Model file for the job. Use its own axes, mm. A direction names the side the tool comes from. Round coordinates to 2 decimals unless told otherwise and drop trailing zeros. Loops run counter-clockwise (first coordinate to the right, second up) from the corner with the lowest first, then second, coordinate; pieces in that order, holes last. Notation, with made-up numbers: (-19, -7.5) - (14, -7.5) arc R30 cw to (14, 20.5) - close; hole circle Ø7 at (-13.75, -18.75). An arc over 180 degrees is marked (long way). Use one line per item in the form item = value.
from build123d import *

# Parameters (mm, degrees)
F1_DEPTH       = 7
F0_R           = 2.75
F2_DEPTH       = 3.175
F3_R           = 12.7
F4_DEPTH       = 6.35
F5_D           = 3.3
F5_CBORE_D     = 6.5
F5_CBORE_DEPTH = 2.5
F6_R           = 5.08
F7_R           = 1.27


with BuildPart() as f1:
    # F0 (on Front) → F1 (new body)
    with BuildSketch(Plane.XZ):
        with BuildLine():
            Line((19.05, 0), (-19.05, 0))
            ThreePointArc((-19.05, 0), (-27.0823171118, -4.4056732068), (-27.6841325359, -13.5471114297))
            Line((-27.6841325359, -13.5471114297), (-8.6341325359, -54.4411114297))
            ThreePointArc((-8.6341325359, -54.4411114297), (0, -59.944), (8.6341325359, -54.4411114297))
            Line((8.6341325359, -54.4411114297), (27.6841325359, -13.5471114297))
            ThreePointArc((27.6841325359, -13.5471114297), (27.0823171118, -4.4056732068), (19.05, 0))
        make_face()
        Polygon((4.9074772881, -50.419), (2.4537386441, -54.669), (-2.4537386441, -54.669), (-4.9074772881, -50.419), (-2.4537386441, -46.169), (2.4537386441, -46.169), align=None, mode=Mode.SUBTRACT)
        Polygon((-14.1425227119, -9.525), (-16.5962613559, -13.775), (-21.5037386441, -13.775), (-23.9574772881, -9.525), (-21.5037386441, -5.275), (-16.5962613559, -5.275), align=None, mode=Mode.SUBTRACT)
        Polygon((23.9574772881, -9.525), (21.5037386441, -13.775), (16.5962613559, -13.775), (14.1425227119, -9.525), (16.5962613559, -5.275), (21.5037386441, -5.275), align=None, mode=Mode.SUBTRACT)
    extrude(amount=F1_DEPTH)

    # F0 (on Front) → F2 (join)
    with BuildSketch(Plane.XZ):
        with BuildLine():
            Line((19.05, 0), (-19.05, 0))
            ThreePointArc((-19.05, 0), (-27.0823171118, -4.4056732068), (-27.6841325359, -13.5471114297))
            Line((-27.6841325359, -13.5471114297), (-8.6341325359, -54.4411114297))
            ThreePointArc((-8.6341325359, -54.4411114297), (0, -59.944), (8.6341325359, -54.4411114297))
            Line((8.6341325359, -54.4411114297), (27.6841325359, -13.5471114297))
            ThreePointArc((27.6841325359, -13.5471114297), (27.0823171118, -4.4056732068), (19.05, 0))
        make_face()
        Polygon((4.9074772881, -50.419), (2.4537386441, -54.669), (-2.4537386441, -54.669), (-4.9074772881, -50.419), (-2.4537386441, -46.169), (2.4537386441, -46.169), align=None, mode=Mode.SUBTRACT)
        Polygon((-14.1425227119, -9.525), (-16.5962613559, -13.775), (-21.5037386441, -13.775), (-23.9574772881, -9.525), (-21.5037386441, -5.275), (-16.5962613559, -5.275), align=None, mode=Mode.SUBTRACT)
        Polygon((23.9574772881, -9.525), (21.5037386441, -13.775), (16.5962613559, -13.775), (14.1425227119, -9.525), (16.5962613559, -5.275), (21.5037386441, -5.275), align=None, mode=Mode.SUBTRACT)
        Polygon((16.5962613559, -13.775), (21.5037386441, -13.775), (23.9574772881, -9.525), (21.5037386441, -5.275), (16.5962613559, -5.275), (14.1425227119, -9.525), align=None)
        with Locations((19.05, -9.525)):
            Circle(F0_R, mode=Mode.SUBTRACT)
        Polygon((-21.5037386441, -13.775), (-16.5962613559, -13.775), (-14.1425227119, -9.525), (-16.5962613559, -5.275), (-21.5037386441, -5.275), (-23.9574772881, -9.525), align=None)
        with Locations((-19.05, -9.525)):
            Circle(F0_R, mode=Mode.SUBTRACT)
        Polygon((-2.4537386441, -54.669), (2.4537386441, -54.669), (4.9074772881, -50.419), (2.4537386441, -46.169), (-2.4537386441, -46.169), (-4.9074772881, -50.419), align=None)
        with Locations((0, -50.419)):
            Circle(F0_R, mode=Mode.SUBTRACT)
    extrude(amount=-F2_DEPTH)

    # F3 (on face) → F4 (join)
    with BuildSketch(Plane(origin=(0, 3.175, 0), x_dir=(-1, 0, 0), z_dir=(0, 1, 0))):
        with BuildLine():
            Line((20.574, -0.1227104384), (20.574, 42.2952895616))
            Line((20.574, 42.2952895616), (-20.574, 42.2952895616))
            Line((-20.574, 42.2952895616), (-20.574, -0.1227104384))
            ThreePointArc((-20.574, -0.1227104384), (-19.8144661294, -0.0307271718), (-19.05, 0))
            Line((-19.05, 0), (19.05, 0))
            ThreePointArc((19.05, 0), (19.8144661294, -0.0307271718), (20.574, -0.1227104384))
        make_face()
        with Locations((0, 21.59)):
            Circle(F3_R, mode=Mode.SUBTRACT)
    extrude(amount=-F4_DEPTH)

    # F5 (through all)
    with Locations(Plane(origin=(0, 3.175, 0), x_dir=(-1, 0, 0), z_dir=(0, 1, 0))):
        with Locations((-15.5, 37.09), (15.5, 37.09), (15.5, 6.09), (-15.5, 6.09)):
            CounterBoreHole(F5_D / 2, F5_CBORE_D / 2, F5_CBORE_DEPTH)

    # F6
    f6_edges = [f1.edges().sort_by_distance(p)[0] for p in [
        (20.574, 0, 42.29529),
        (-20.574, 0, 42.29529),
        (-20.574, 0, -0.12271),
        (20.574, 0, -0.12271),
    ]]
    fillet(f6_edges, radius=F6_R)

    # F7
    f7_edges = [f1.edges().sort_by_distance(p)[0] for p in [
        (28.052301, 3.175, -6.413054),
        (18.159133, -7, -33.994111),
    ]]
    fillet(f7_edges, radius=F7_R)


solid = f1.part
1. Tool access for faces 4 (the flat face through (20.574, -1, 21)), 5 (the cylindrical face through (-12.921, 1.942, 4.112)), 6 (the flat face through (-22.7, -3.5, -11.7)), 7 (the flat face through (0, 3.175, -8)), 8 (the cylindrical face through (17.95, 2.81, -33.55)): list every direction of +Z, -Z, +X, -X, +Y, -Y with a clear straight run to the whole face (end or side of a thin tool).
Geometry check:
face_4 = +Z, +X, +Y, -Y
face_5 = +Y
face_6 = -Y
face_7 = +Z, -Z, +X, -X, +Y
face_8 = -Z, +X, +Y
2. Cut at A-A, the plane z = 21.59. Give the cut face in (x, y) (3 decimals), plus the area to 3 significant figures.
Geometry check:
outline = (-20.574, -3.175) - (-12.7, -3.175) - (-12.7, 3.175) - (-19.304, 3.175) arc R1.27 ccw to (-20.574, 1.905) - close; (12.7, -3.175) - (20.574, -3.175) - (20.574, 1.905) arc R1.27 ccw to (19.304, 3.175) - (12.7, 3.175) - close
area = 99.3 mm^2
3. Pull direction Z, two halves, no side cores. Call faces 1 (the flat face through (15.4, -3.5, -11.7)), 2 (the cylindrical face through (-21.305, -0.671, 0.876)), 3 (the flat face through (-20.574, -1, 20)): +Z half, -Z half, draft (parallel to the pull), parting line (faces both ways), or undercut.
Geometry check:
face_1 = undercut
face_2 = +Z half
face_3 = draft
4. Wall check: probe 1 along X at (y, z) = (-5.25, -9.5); probe 2 along X at (y, z) = (-3.5, -10.5); probe 3 along Z at (x, y) = (15.5, 2.05). Give the ranges that are in metal, low to high.
Geometry check:
probe_1 = -28.57 to -23.94, -14.16 to 14.16, 23.94 to 28.57
probe_2 = -28.52 to -23.39, -14.71 to 14.71, 23.39 to 28.52
probe_3 = -39.68 to 2.84, 9.34 to 33.84, 40.34 to 42.29
5. Flat gauge pins, fed straight in: pin 1 (1.5 mm diameter, centred on x = -20, y = -5, fed in from -Z); pin 2 (2 mm diameter, centred on x = 15.5, z = 6.09, fed in from +Y); pin 3 (1 mm diameter, centred on x = -14.5, y = -3.5, fed in from -Z); pin 4 (3 mm diameter, centred on x = -15, z = 37, fed in from +Y) (3 decimals). Where does each tip first touch, or does it go through?
Geometry check:
pin_1 = -31.65
pin_2 = through
pin_3 = -42.92
pin_4 = 0.675
6. Cut at B-B, the plane z = 6.09. Give the cut face in (x, y) (3 decimals), plus the area to 3 significant figures.
Geometry check:
outline = (-20.574, -3.175) - (-17.15, -3.175) - (-17.15, 0.675) - (-18.75, 0.675) - (-18.75, 3.175) - (-19.304, 3.175) arc R1.27 ccw to (-20.574, 1.905) - close; (-13.85, -3.175) - (13.85, -3.175) - (13.85, 0.675) - (12.25, 0.675) - (12.25, 3.175) - (-12.25, 3.175) - (-12.25, 0.675) - (-13.85, 0.675) - close; (17.15, -3.175) - (20.574, -3.175) - (20.574, 1.905) arc R1.27 ccw to (19.304, 3.175) - (18.75, 3.175) - (18.75, 0.675) - (17.15, 0.675) - close
area = 203 mm^2
